from build123d import *

# Parameters (mm, degrees)
SKETCH1_R           = 1.778
BOSS_EXTRUDE1_DEPTH = 6.35


with BuildPart() as part:
    # Sketch1 → Boss-Extrude1 (new body)
    with BuildSketch(Plane.XZ):
        with BuildLine():
            Line((-29.337, -4.7625), (29.337, -4.7625))
            ThreePointArc((29.337, -4.7625), (34.0995, 0), (29.337, 4.7625))
            Line((29.337, 4.7625), (-29.337, 4.7625))
            ThreePointArc((-29.337, 4.7625), (-34.0995, 0), (-29.337, -4.7625))
        make_face()
        with Locations(Location((29.337, 0, 0), (0, 0, 90))):
            Circle(SKETCH1_R, mode=Mode.SUBTRACT)
        with Locations(Location((19.558, 0, 0), (0, 0, 90))):
            Circle(SKETCH1_R, mode=Mode.SUBTRACT)
        with Locations(Location((9.779, 0, 0), (0, 0, 90))):
            Circle(SKETCH1_R, mode=Mode.SUBTRACT)
        with Locations(Location((0, 0, 0), (0, 0, 90))):
            Circle(SKETCH1_R, mode=Mode.SUBTRACT)
        with Locations(Location((-9.779, 0, 0), (0, 0, 90))):
            Circle(SKETCH1_R, mode=Mode.SUBTRACT)
        with Locations(Location((-19.558, 0, 0), (0, 0, 90))):
            Circle(SKETCH1_R, mode=Mode.SUBTRACT)
        with Locations(Location((-29.337, 0, 0), (0, 0, 90))):
            Circle(SKETCH1_R, mode=Mode.SUBTRACT)
    extrude(amount=-BOSS_EXTRUDE1_DEPTH)


solid = part.part
Input: part model. Units: mm. Frame: model coordinates. Give positions to 0.01 mm unless a question says otherwise; leave off trailing zeros. Write each loop counter-clockwise with the first axis right and the second up, starting at its lowest first coordinate (ties: lowest second). Pieces come first, ordered by that corner, then holes. Notation, with made-up numbers: (-16.75, -3) -> (34.25, -3) arc R24 ccw to (34.25, 35) -> close; hole circle Ø1 at (8.5, -26). An arc over 180 degrees is marked (long way). Use one line per item in the form item = value. Start each with the question number.
1) Section query D-D on x = -10.5. Return the cut outline in (y, z).
2) Ray query, probe 1 along Z at (x, y) = (-18.5, 5.5); probe 2 along Z at (x, y) = (21, 6); probe 3 along X at (y, z) = (5, -2). Return the intervals inside material, ascending. Write a range as from..to.
3) Draft query along Z for faces 1 (the cylindrical face through (1.736, 3.131, -0.385)), 2 (the cylindrical face through (-34.1, 3.1, 0.1)), 3 (the flat face through (0, 0, 2)). Return one class per face: pulls with the +Z half, pulls with the -Z half, needs draft (parallel to the pull), parting line crosses it, or undercut.
4) Section query B-B on x = 0. Return the cut outline in (y, z), then the cut area to 3 significant figures.
5) Section query A-A on z = 0. Count the separate pieces of the cut face and the enclosed holes in it, then the cut area to 3 significant figures.
6) Section query C-C on y = 5. Return the cut outline in (x, z) (1 decimal), then the cut area to 3 significant figures.
Outcome:
q1.outline = (0, -4.76) -> (6.35, -4.76) -> (6.35, -1.63) -> (0, -1.63) -> close; (0, 1.63) -> (6.35, 1.63) -> (6.35, 4.76) -> (0, 4.76) -> close
q2.probe_1 = -4.76..-1.43, 1.43..4.76
q2.probe_2 = -4.76..-1.04, 1.04..4.76
q2.probe_3 = -33.66..33.66
q3.face_1 = undercut
q3.face_2 = parting line crosses it
q3.face_3 = needs draft
q4.outline = (0, -4.76) -> (6.35, -4.76) -> (6.35, -1.78) -> (0, -1.78) -> close; (0, 1.78) -> (6.35, 1.78) -> (6.35, 4.76) -> (0, 4.76) -> close
q4.area = 37.9 mm^2
q5.separate_pieces = 8
q5.enclosed_holes = 0
q5.area = 275 mm^2
q6.outline = (-29.3, -4.8) -> (29.3, -4.8) arc R4.8 ccw to (29.3, 4.8) -> (-29.3, 4.8) arc R4.8 ccw to start; hole circle Ø3.6 at (-29.3, 0); hole circle Ø3.6 at (-19.6, 0); hole circle Ø3.6 at (-9.8, 0); hole circle Ø3.6 at (0, 0); hole circle Ø3.6 at (9.8, 0); hole circle Ø3.6 at (19.6, 0); hole circle Ø3.6 at (29.3, 0)
q6.area = 561 mm^2
